```python
from build123d import *

# Parameters (mm, degrees)
F0_R     = 41.5439468533
F1_DEPTH = 15
F2_SIZE  = 5
F3_T     = -2
F4_R     = 1


with BuildPart() as f1:
    # F0 (on Top) → F1 (new body)
    with BuildSketch(Plane.XY):
        Circle(F0_R)
    extrude(amount=F1_DEPTH)

    # F2
    f2_edges = [f1.edges().sort_by_distance(p)[0] for p in [
        (-41.543947, 0, 15),
    ]]
    chamfer(f2_edges, length=F2_SIZE)

    # F3
    f3_openings = [f1.faces().sort_by_distance(p)[0] for p in [
        (0, 0, 0),
    ]]
    offset(amount=F3_T, openings=f3_openings)

    # F4
    f4_edges = [f1.edges().sort_by_distance(p)[0] for p in [
        (39.043947, 0, 12.5),
        (-41.543947, 0, 10),
        (-36.543947, 0, 15),
    ]]
    fillet(f4_edges, radius=F4_R)


solid = f1.part
```
CAD build for the part. Positions are in the model's coordinates, mm. A direction names the side the tool comes from. Coordinates: 2 decimals unless noted, no trailing zeros. Order: outer loops, then holes, each group sorted by start corner. A loop starts at its lowest first (then second) coordinate and runs counter-clockwise, first axis right, second up.
(1) Which spindle directions (+Z, -Z, +X, -X, +Y, -Y) get a long thin tool onto all of the face, cutting with end or side? Do faces 1 (the face through (35.34, 11.13, 14.49)), 2 (the face through (-1, 1, 13)). Say none if no direction does.
Solution:
face 1: +Z
face 2: -Z
(2) Drill centre lines: L1, parallel to Y at x = 0, z = 3; L2, parallel to X at y = -30, z = 9.25. Where is each one in solid material? Low to high.
Solution:
L1: y = -41.54 to -39.54, 39.54 to 41.54
L2: x = -28.74 to -25.64, 25.64 to 28.74
(3) Saw through at A-A, the plane z = 6.25. Write the cut outline in (x, y).
Solution:
outline: circle Ø83.09 at (0, 0); hole circle Ø79.09 at (0, 0)
(4) Mould opens along X. For faces 3 (the face through (-1, 1, 15)), 4 (the face through (-29.146, 26.726, 4.522)), 5 (the face through (19.17, -36.857, 4.726)) say: released by +X, released by -X, zero draft, split by the parting line, or undercut.
Solution:
face 3: zero draft
face 4: undercut
face 5: split by the parting line
(5) Pin check, flat tips, straight feed: pin 1 Ø2 at (y, z) = (-3, 9) entering from +X; pin 2 Ø2 at (y, z) = (-8.5, 4.5) entering from +X; pin 3 Ø6 at (y, z) = (-14, 11.5) entering from +X. Stop position of each tip, or through.
Solution:
pin 1: stops at x = 41.5
pin 2: stops at x = 40.86
pin 3: stops at x = 39.89
